```python
from build123d import *

# Parameters (mm, degrees)
SKETCH1_R            = 67.5
BOSS_EXTRUDE1_DEPTH  = 21
SKETCH3_R            = 80
BOSS_EXTRUDE2_DEPTH  = 25
SKETCH4_R            = 87.5
BOSS_EXTRUDE3_DEPTH  = 4
SHELL1_START         = 4
SHELL1_OUTLINE_R     = 63.5
SHELL1_DEPTH         = 46
SHELL1_START_2       = 25
SHELL1_2_OUTLINE_R   = 76
SHELL1_2_OUTLINE_R_2 = 63.5
SHELL1_2_DEPTH       = 25
SKETCH2_R            = 11
SKETCH2_R_2          = 6.25
CUT_EXTRUDE1_DEPTH   = 10
SKETCH5_R            = 15
SKETCH5_R_2          = 6.25
BOSS_EXTRUDE4_DEPTH  = 20
SKETCH6_R            = 12.5
CUT_EXTRUDE2_DEPTH   = 20
CHAMFER1_SIZE        = 3
CHAMFER2_SIZE        = 3
SKETCH7_R            = 15
SKETCH7_R_2          = 11
BOSS_EXTRUDE5_DEPTH  = 5


# Read off the part's stored shape, not the designer's step: Shell1
with BuildPart() as part:
    # Sketch1 → Boss-Extrude1 (new body)
    with BuildSketch(Plane(origin=(0, 0, 0), x_dir=(1, 0, 0), z_dir=(0, 1, 0))):
        with Locations(Location((0, 0, 0), (0, 0, 90))):
            Circle(SKETCH1_R)
    extrude(amount=BOSS_EXTRUDE1_DEPTH)

    # Sketch3 → Boss-Extrude2 (add)
    with BuildSketch(Plane(origin=(0, 21, 0), x_dir=(1, 0, 0), z_dir=(0, 1, 0))):
        with Locations(Location((0, 0, 0), (0, 0, 270))):
            Circle(SKETCH3_R)
    extrude(amount=BOSS_EXTRUDE2_DEPTH)

    # Sketch4 → Boss-Extrude3 (add)
    with BuildSketch(Plane(origin=(0, 46, 0), x_dir=(1, 0, 0), z_dir=(0, 1, 0))):
        with Locations(Location((0, 0, 0), (0, 0, 270))):
            Circle(SKETCH4_R)
    extrude(amount=BOSS_EXTRUDE3_DEPTH)

    # Shell1 outline → Shell1 (cut)
    with BuildSketch(Plane(origin=(0, 0, 0), x_dir=(1, 0, 0), z_dir=(0, 1, 0)).offset(SHELL1_START)):
        Circle(SHELL1_OUTLINE_R)
    extrude(amount=SHELL1_DEPTH, mode=Mode.SUBTRACT)

    # Shell1 2 outline → Shell1 2 (cut)
    with BuildSketch(Plane(origin=(0, 0, 0), x_dir=(1, 0, 0), z_dir=(0, 1, 0)).offset(SHELL1_START_2)):
        Circle(SHELL1_2_OUTLINE_R)
        Circle(SHELL1_2_OUTLINE_R_2, mode=Mode.SUBTRACT)
    extrude(amount=SHELL1_2_DEPTH, mode=Mode.SUBTRACT)

    # Sketch2 → Cut-Extrude1 (cut)
    with BuildSketch(Plane(origin=(0, 4, 0), x_dir=(1, 0, 0), z_dir=(0, 1, 0))):
        with Locations(Location((0, 22.5, 0), (0, 0, 270))):
            Circle(SKETCH2_R)
        with Locations(Location((-35, 22.5, 0), (0, 0, 270))):
            Circle(SKETCH2_R_2)
        with Locations(Location((35, 22.5, 0), (0, 0, 270))):
            Circle(SKETCH2_R_2)
    extrude(amount=-CUT_EXTRUDE1_DEPTH, mode=Mode.SUBTRACT)

    # Sketch5 → Boss-Extrude4 (add)
    # profile 1 of 2: a face of its own
    with BuildSketch(Plane.XZ):
        with Locations(Location((35, -22.5, 0), (0, 0, 90))):
            Circle(SKETCH5_R)
        with Locations(Location((35, -22.5, 0), (0, 0, 90))):
            Circle(SKETCH5_R_2, mode=Mode.SUBTRACT)
    # profile 2 of 2: a face of its own
    with BuildSketch(Plane.XZ):
        with Locations(Location((-35, -22.5, 0), (0, 0, 90))):
            Circle(SKETCH5_R)
        with Locations(Location((-35, -22.5, 0), (0, 0, 90))):
            Circle(SKETCH5_R_2, mode=Mode.SUBTRACT)
    extrude(amount=BOSS_EXTRUDE4_DEPTH)

    # Sketch6 → Cut-Extrude2 (cut)
    with BuildSketch(Plane(origin=(0, 4, 0), x_dir=(1, 0, 0), z_dir=(0, 1, 0))):
        with Locations(Location((-35, 22.5, 0), (0, 0, 270))):
            Circle(SKETCH6_R)
        with Locations(Location((35, 22.5, 0), (0, 0, 270))):
            Circle(SKETCH6_R)
    extrude(amount=-CUT_EXTRUDE2_DEPTH, mode=Mode.SUBTRACT)

    # Chamfer1
    chamfer1_edges = [part.edges().sort_by_distance(p)[0] for p in [
        (0, 0, 67.5),
        (0, 21, -80),
    ]]
    chamfer(chamfer1_edges, length=CHAMFER1_SIZE)

    # Chamfer2
    chamfer2_edges = [part.edges().sort_by_distance(p)[0] for p in [
        (35, -20, -37.5),
        (-35, -20, -37.5),
    ]]
    chamfer(chamfer2_edges, length=CHAMFER2_SIZE)

    # Sketch7 → Boss-Extrude5 (add)
    with BuildSketch(Plane.XZ):
        with Locations(Location((0, -22.5, 0), (0, 0, 90))):
            Circle(SKETCH7_R)
        with Locations(Location((0, -22.5, 0), (0, 0, 90))):
            Circle(SKETCH7_R_2, mode=Mode.SUBTRACT)
    extrude(amount=BOSS_EXTRUDE5_DEPTH)


solid = part.part
```
Design review of the part built by this model. Coordinates are the model's own, in mm. A direction names the side the tool comes from. Give positions to 0.01 mm unless a question says otherwise; leave off trailing zeros. Order: outer loops, then holes, each group sorted by start corner. A loop starts at its lowest first (then second) coordinate and runs counter-clockwise, first axis right, second up. Notation, with made-up numbers: (19, 25.5) -> (35, 25.5) arc R32 cw to (35, 61.5) -> close; hole circle Ø1 at (75.25, 28.5). An arc over 180 degrees is marked (long way). Write item = value, one per line. Start each with the question number.
(1) We need section B-B on y = -13. Write out the cut boundary in (x, z).
(2) We need section C-C on z = -22.5. State how many separate pieces and enclosed holes the cut face has, plus the area to 3 significant figures.
(3) To check wall thickness, follow line 1 along X through (y, z) = (13.75, 0); line 2 along X through (y, z) = (28.5, 0); line 3 along X through (y, z) = (-19.2, -22.5). State the ranges of each line that lie inside material, in increasing order.
(4) We need section D-D on y = 41. Write out the cut boundary in (x, z).
(5) For faces 1 (the face through (86.755, 47.972, -11.391)), 2 (the face through (-68, 21, 0)), 3 (the face through (-1, 4, -1)), list the 3-axis set-ups (+Z, -Z, +X, -X, +Y, -Y) from which the entire face can be reached by the end or side of a thin tool; tool diameter is ignored.
(6) For pin 1 (14.5 mm diameter, centred on x = 35, z = -22.5, fed in from +Y); pin 2 (6 mm diameter, centred on x = -2.5, y = -4.5, fed in from +Z); pin 3 (10 mm diameter, centred on x = -34, y = 35, fed in from +Z), all flat-tipped, find the tip position at first contact; note any pin that passes through.
(7) Mouldability with a two-part tool opening along Z and no side actions: class faces 4 (the face through (-11.2, -5, -23.7)), 5 (the face through (35.069, 37.325, 67.425)), 6 (the face through (20.128, -8.381, -24.453)) as +Z half, -Z half, draft (parallel to the pull), parting line (faces both ways), or undercut.
Numbers:
q1.outline = circle Ø30 at (-35, -22.5); circle Ø30 at (35, -22.5); hole circle Ø25 at (-35, -22.5); hole circle Ø25 at (35, -22.5)
q2.separate_pieces = 4
q2.enclosed_holes = 0
q2.area = 1,080 mm^2
q3.line_1 = -67.5 to -63.5, 63.5 to 67.5
q3.line_2 = -80 to -76, 76 to 80
q3.line_3 = -47.8 to -41.25, -28.75 to -22.2, 22.2 to 28.75, 41.25 to 47.8
q4.outline = circle Ø160 at (0, 0); hole circle Ø152 at (0, 0)
q5.face_1 = +Y, -Y
q5.face_2 = -Y
q5.face_3 = +Y
q6.pin_1 = -16
q6.pin_2 = -7.5
q6.pin_3 = 74.56
q7.face_4 = draft
q7.face_5 = undercut
q7.face_6 = parting line
